Can you work these out from the model? Positions are in its coordinate system, mm. Face numbers are marked on the shaded views. Give positions to 0.01 mm unless a question says otherwise; leave off trailing zeros. Write each loop counter-clockwise with the first axis right and the second up, starting at its lowest first coordinate (ties: lowest second). Pieces come first, ordered by that corner, then holes.
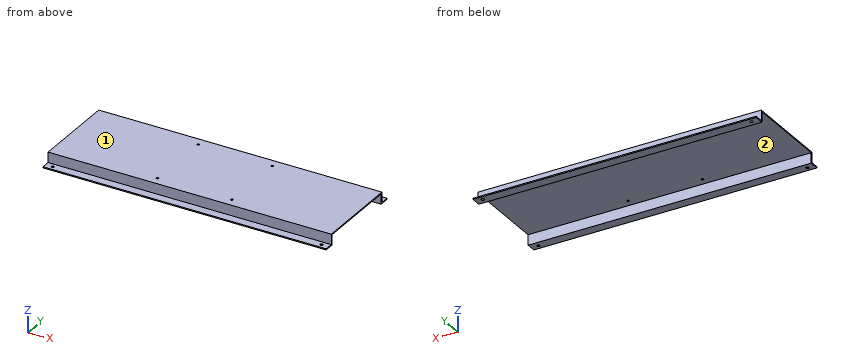
```python
from build123d import *

# Parameters (mm, degrees)
F1_DEPTH = 314.325
F2_R     = 2.579688
F2_R_2   = 3.175
F3_DEPTH = 25.401


with BuildPart() as f1:
    # F0 (on Right) → F1 (new body, symmetric)
    with BuildSketch(Plane.YZ):
        Polygon((-114.3, 2.54), (-114.3, 0), (-92.6338, 0), (-92.6338, 22.86), (92.6338, 22.86), (92.6338, 0), (114.3, 0), (114.3, 2.54), (95.1738, 2.54), (95.1738, 25.4), (-95.1738, 25.4), (-95.1738, 2.54), align=None)
    extrude(amount=F1_DEPTH, both=True)

    # F2 (on face) → F3 (cut, through all)
    with BuildSketch(Plane.XY.offset(25.4)):
        with Locations((-82.55, 76.2)):
            Circle(F2_R)
        with Locations((-82.55, -76.2)):
            Circle(F2_R)
        with Locations((82.55, -76.2)):
            Circle(F2_R)
        with Locations((82.55, 76.2)):
            Circle(F2_R)
        with Locations((298.45, 104.775)):
            Circle(F2_R_2)
        with Locations((298.45, -104.775)):
            Circle(F2_R_2)
        with Locations((-298.45, -104.775)):
            Circle(F2_R_2)
        with Locations((-298.45, 104.775)):
            Circle(F2_R_2)
    extrude(amount=-F3_DEPTH, mode=Mode.SUBTRACT)


solid = f1.part
```
1) Suppose I cut it at C-C on y = 16. Write out the boundary of the cut face in (x, z) (3 decimals).
Values follow:
outline: (-314.325, 22.86) - (314.325, 22.86) - (314.325, 25.4) - (-314.325, 25.4) - close
2) For pin 1 Ø15.5 at (x, y) = (-82, 102.5) entering from +Z; pin 2 Ø8.5 at (x, y) = (82.55, -76.2) entering from -Z; pin 3 Ø1 at (x, z) = (151, 22.5) entering from +Y; pin 4 Ø12 at (y, z) = (-82.5, 10.5) entering from +X, each with a flat end and sliding along its axis, tell me the tip position at first contact or that it passes through.
Values follow:
pin 1: stops at z = 25.4
pin 2: stops at z = 22.86
pin 3: stops at y = 95.17
pin 4: passes through
3) Please list where these lines run through material, in increasing order: L1, parallel to Y at x = 82.55, z = 24.05; L2, parallel to Y at x = -298.45, z = 1.5; L3, parallel to Y at x = -115, z = 13.
Values follow:
L1: y = -95.17 to -78.78, -73.62 to 73.62, 78.78 to 95.17
L2: y = -114.3 to -107.95, -101.6 to -92.63, 92.63 to 101.6, 107.95 to 114.3
L3: y = -95.17 to -92.63, 92.63 to 95.17
4) Suppose I cut it at A-A on z = 6.5. Write out the boundary of the cut face in (x, y) (3 decimals), plus the area to 3 significant figures.
Values follow:
outline: (-314.325, -95.174) - (314.325, -95.174) - (314.325, -92.634) - (-314.325, -92.634) - close; (-314.325, 92.634) - (314.325, 92.634) - (314.325, 95.174) - (-314.325, 95.174) - close
area: 3,190 mm2
5) Suppose I cut it at B-B on x = 115.5. Write out the boundary of the cut face in (y, z).
Values follow:
outline: (-114.3, 0) - (-92.63, 0) - (-92.63, 22.86) - (92.63, 22.86) - (92.63, 0) - (114.3, 0) - (114.3, 2.54) - (95.17, 2.54) - (95.17, 25.4) - (-95.17, 25.4) - (-95.17, 2.54) - (-114.3, 2.54) - close
6) If we mould it in two halves opening along Y, with no side actions, what happens to the marked faces 1 and 2? For each: +Y half, -Y half, draft (parallel to the pull), parting line (faces both ways), or undercut.
Values follow:
face 1: draft
face 2: undercut
